```python
from build123d import *

# Parameters (mm, degrees)
F0_W     = 40
F0_H     = 20
F0_R     = 1.6
F0_R_2   = 6.25
F1_DEPTH = 11
F2_R     = 9
F2_R_2   = 6.2
F3_DEPTH = 8
F4_R     = 5


with BuildPart() as f1:
    # F0 (on Top) → F1 (new body)
    with BuildSketch(Plane.XY):
        with Locations((20, 10)):
            Rectangle(F0_W, F0_H)
        with Locations((8, 10)):
            Circle(F0_R, mode=Mode.SUBTRACT)
        with Locations((20, 10)):
            Circle(F0_R_2, mode=Mode.SUBTRACT)
        with Locations((32, 10)):
            Circle(F0_R, mode=Mode.SUBTRACT)
    extrude(amount=F1_DEPTH)

    # F2 (on face) → F3 (join)
    with BuildSketch(Plane.XY.offset(11)):
        with Locations((20, 10)):
            Circle(F2_R)
        with Locations((20, 10)):
            Circle(F2_R_2, mode=Mode.SUBTRACT)
    extrude(amount=F3_DEPTH)

    # F4
    f4_edges = [f1.edges().sort_by_distance(p)[0] for p in [
        (40, 20, 5.5),
        (40, 0, 5.5),
        (0, 0, 5.5),
        (0, 20, 5.5),
    ]]
    fillet(f4_edges, radius=F4_R)


solid = f1.part
```
The model under review builds one solid part; all positions refer to its coordinate system, in mm. A direction names the side the tool comes from. Give positions to 0.01 mm unless a question says otherwise; leave off trailing zeros. Write each loop counter-clockwise with the first axis right and the second up, starting at its lowest first coordinate (ties: lowest second). Pieces come first, ordered by that corner, then holes.
(1) The part is to be moulded in two halves that separate along X. For faces 3 (the cylindrical face through (15.04, 6.2, 5.42)), 4 (the flat face through (40, 10, 5)), 5 (the flat face through (21.9, 16.1, 19)), say which applies: released by +X, released by -X, zero draft, split by the parting line, or undercut.
(2) To check wall thickness, follow L1, parallel to Y at x = 20, z = 14; L2, parallel to Z at x = 34, y = 11.5; L3, parallel to Y at x = 20, z = 3. State the ranges of each line that lie inside material, in increasing order.
(3) Consider section A-A, the plane y = 10. Give the boundary of the cut face in (x, z), and give its area (3 significant figures).
(4) For P1, Ø11, axis at x = 20, y = 10, coming from the +Z side; P2, Ø6, axis at x = 21, y = 15, coming from the -Z side; P3, Ø5, axis at x = 32, y = 10, coming from the +Z side; P4, Ø3, axis at y = 10.5, z = 17, coming from the +X side, all flat-tipped, find the tip position at first contact; note any pin that passes through.
(5) Consider section D-D, the plane y = 8. Give the boundary of the cut face in (x, z).
(6) Consider section C-C, the plane z = 6.25. Give the boundary of the cut face in (x, y).
(7) Tool access review of faces 1 (the cylindrical face through (28.314, 6.553, 14.944)), 2 (the flat face through (15, 6, 0)): name each direction out of +Z, -Z, +X, -X, +Y, -Y from which nothing blocks a thin tool from reaching the whole face with its end or side.
(8) Consider section B-B, the plane x = 20. Give the boundary of the cut face in (y, z), and give its area (3 significant figures).
Returned:
1. face 3: undercut
1. face 4: released by +X
1. face 5: zero draft
2. L1: y = 1 to 3.8, 16.2 to 19
2. L2: z = 0 to 11
2. L3: y = 0 to 3.75, 16.25 to 20
3. outline: (0, 0) - (6.4, 0) - (6.4, 11) - (0, 11) - close; (9.6, 0) - (13.75, 0) - (13.75, 11) - (13.8, 11) - (13.8, 19) - (11, 19) - (11, 11) - (9.6, 11) - close; (26.2, 11) - (26.25, 11) - (26.25, 0) - (30.4, 0) - (30.4, 11) - (29, 11) - (29, 19) - (26.2, 19) - close; (33.6, 0) - (40, 0) - (40, 11) - (33.6, 11) - close
3. area: 277 mm2
4. P1: passes through
4. P2: stops at z = 0
4. P3: stops at z = 11
4. P4: stops at x = 29
5. outline: (0, 0) - (14.08, 0) - (14.08, 11) - (14.13, 11) - (14.13, 19) - (11.23, 19) - (11.23, 11) - (0, 11) - close; (25.87, 11) - (25.92, 11) - (25.92, 0) - (40, 0) - (40, 11) - (28.77, 11) - (28.77, 19) - (25.87, 19) - close
6. outline: (0, 5) arc R5 ccw to (5, 0) - (35, 0) arc R5 ccw to (40, 5) - (40, 15) arc R5 ccw to (35, 20) - (5, 20) arc R5 ccw to (0, 15) - close; hole circle Ø3.2 at (8, 10); hole circle Ø12.5 at (20, 10); hole circle Ø3.2 at (32, 10)
7. face 1: +Z
7. face 2: -Z, +X, -X, +Y, -Y
8. outline: (0, 0) - (3.75, 0) - (3.75, 11) - (3.8, 11) - (3.8, 19) - (1, 19) - (1, 11) - (0, 11) - close; (16.2, 11) - (16.25, 11) - (16.25, 0) - (20, 0) - (20, 11) - (19, 11) - (19, 19) - (16.2, 19) - close
8. area: 127 mm2
